```python
from build123d import *

# Parameters (mm, degrees)
SKETCH1_R           = 7.5
BOSS_EXTRUDE1_DEPTH = 50
CHAMFER1_SIZE       = 5
CHAMFER2_SIZE       = 2


with BuildPart() as part:
    # Sketch1 → Boss-Extrude1 (new body)
    with BuildSketch(Plane(origin=(0, 0, 0), x_dir=(1, 0, 0), z_dir=(0, 1, 0))):
        with Locations(Location((0, 0, 0), (0, 0, 270))):
            Circle(SKETCH1_R)
    extrude(amount=BOSS_EXTRUDE1_DEPTH)

    # Chamfer1
    chamfer1_edges = [part.edges().sort_by_distance(p)[0] for p in [
        (0, 0, -7.5),
    ]]
    chamfer(chamfer1_edges, length=CHAMFER1_SIZE)

    # Chamfer2
    chamfer2_edges = [part.edges().sort_by_distance(p)[0] for p in [
        (0, 50, -7.5),
    ]]
    chamfer(chamfer2_edges, length=CHAMFER2_SIZE)

    # Sketch2 → Cut-Revolve1 (revolve, cut)
    with BuildSketch(Plane.XY, mode=Mode.PRIVATE) as cut_revolve1_sk:
        Polygon((7.5, 36.190061777), (5.908616691, 33.28526698), (5.908616691, 30.776580564), (4.081049732, 27.440673393), (4.522237355, 22.854412934), (5.908616691, 19.421473627), (5.215427023, 16.71473302), (5.908616691, 12.753649205), (5.22558542, 10.08657472), (7.5, 7.208131864), (18.320012644, 16.71473302), align=None)
    revolve(cut_revolve1_sk.sketch.rotate(Axis((0, 0, 0), (0, 1, 0)), 90), axis=Axis((0, 0, 0), (0, 1, 0)), mode=Mode.SUBTRACT)


solid = part.part
```
Read the model definition and answer for the solid it produces. Units are mm, in the model's axes. A direction names the side the tool comes from. Give positions to 0.01 mm unless a question says otherwise; leave off trailing zeros. Loops run counter-clockwise (first coordinate to the right, second up) from the corner with the lowest first, then second, coordinate; pieces in that order, holes last.
Item 1: The mould has two halves that part along Y. Classify faces 3 (the conical face through (-1.28, 25.63, -4.06)), 4 (the cylindrical face through (0.33, 42.012, -7.493)), 5 (the flat face through (0, 0, 0)), 6 (the cylindrical face through (-1.775, 32.013, -5.636)): released by +Y, released by -Y, zero draft, split by the parting line, or undercut.
Item 2: Find the intervals of material crossed by line 1 along Y through (x, z) = (-4.5, 5.25); line 2 along Y through (x, z) = (-4.5, -2.5); line 3 along Z through (x, y) = (-0.75, 46), in increasing order.
Item 3: The part is cut by section C-C (z = 0). Write down the section's boundary in (x, y).
Item 4: The part is cut by section D-D (y = 29). Write down the section's boundary in (x, z), and give its area (3 significant figures).
Item 5: The part is cut by section B-B (x = 0). Write down the section's boundary in (y, z), and give its area (3 significant figures).
Item 6: For faces 1 (the conical face through (-3.658, 15.587, 3.989)), 2 (the flat face through (0, 50, 0)), determine the directions among +Z, -Z, +X, -X, +Y, -Y from which every point of the face is accessible in a straight line to the end or side of a thin tool.
Item 7: The part is cut by section A-A (y = 43.5). Write down the section's boundary in (x, z).
Item 8: Each of these flat-tipped pins is pushed along its axis until it touches: pin 1 Ø5 at (x, y) = (4, 6) entering from -Z; pin 2 Ø3 at (y, z) = (21, 5) entering from +X; pin 3 Ø2 at (x, z) = (4, -5) entering from -Y. Where does it stop, or does it pass through?
Taken from the geometry:
1. face 3: undercut
1. face 4: zero draft
1. face 5: released by -Y
1. face 6: undercut
2. line 1: y = 4.41 to 7.95, 35.12 to 48.59
2. line 2: y = 2.65 to 21.31, 29.39 to 50
2. line 3: z = -7.46 to 7.46
3. outline: (-7.5, 5) - (-2.5, 0) - (2.5, 0) - (7.5, 5) - (7.5, 7.21) - (5.23, 10.09) - (5.91, 12.75) - (5.22, 16.71) - (5.91, 19.42) - (4.52, 22.85) - (4.08, 27.44) - (5.91, 30.78) - (5.91, 33.29) - (7.5, 36.19) - (7.5, 48) - (5.5, 50) - (-5.5, 50) - (-7.5, 48) - (-7.5, 36.19) - (-5.91, 33.29) - (-5.91, 30.78) - (-4.08, 27.44) - (-4.52, 22.85) - (-5.91, 19.42) - (-5.22, 16.71) - (-5.91, 12.75) - (-5.23, 10.09) - (-7.5, 7.21) - close
4. outline: circle Ø9.87 at (0, 0)
4. area: 76.5 mm2
5. outline: (0, -2.5) - (5, -7.5) - (7.21, -7.5) - (10.09, -5.23) - (12.75, -5.91) - (16.71, -5.22) - (19.42, -5.91) - (22.85, -4.52) - (27.44, -4.08) - (30.78, -5.91) - (33.29, -5.91) - (36.19, -7.5) - (48, -7.5) - (50, -5.5) - (50, 5.5) - (48, 7.5) - (36.19, 7.5) - (33.29, 5.91) - (30.78, 5.91) - (27.44, 4.08) - (22.85, 4.52) - (19.42, 5.91) - (16.71, 5.22) - (12.75, 5.91) - (10.09, 5.23) - (7.21, 7.5) - (5, 7.5) - (0, 2.5) - close
5. area: 604 mm2
6. face 1: none
6. face 2: +Z, -Z, +X, -X, +Y
7. outline: circle Ø15 at (0, 0)
8. pin 1: stops at z = -7.35
8. pin 2: stops at x = 4.17
8. pin 3: stops at y = 2.9
